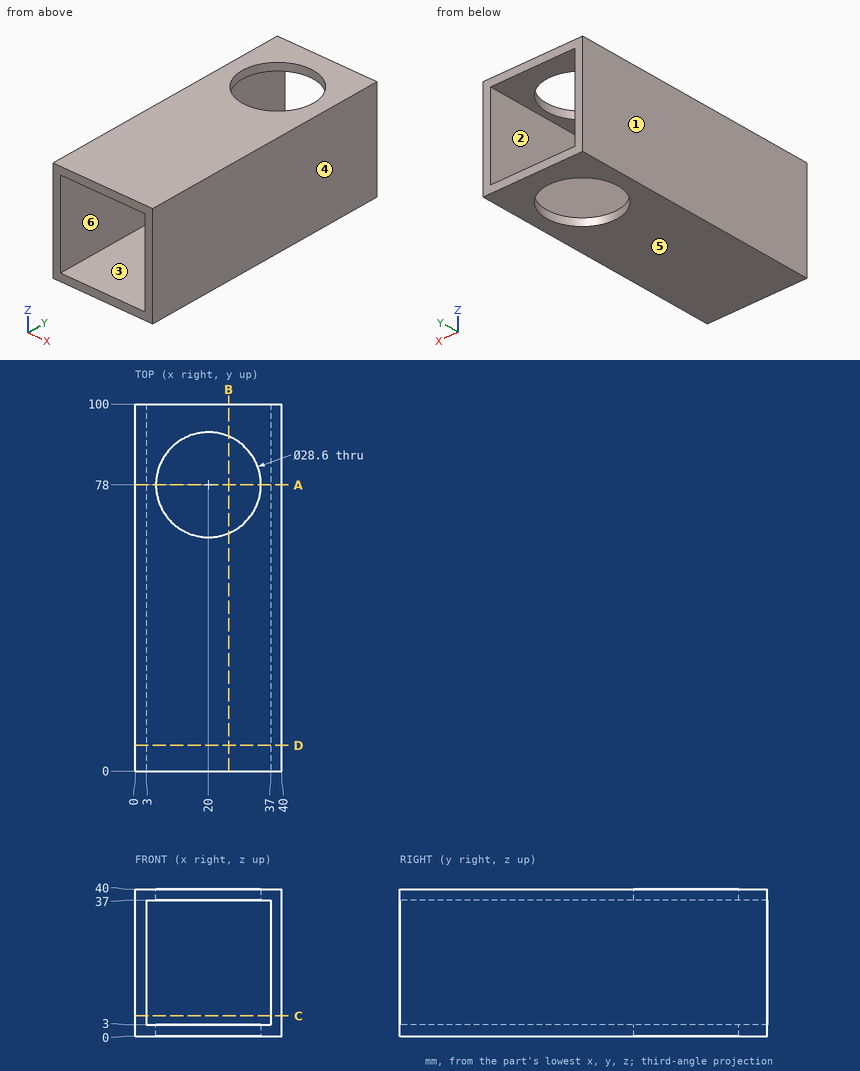
Check sheet for the drawn part. Datum: minimum x, y, z corner. Units: mm. A direction names the side the tool comes from. Round coordinates to 2 decimals unless told otherwise and drop trailing zeros. Order: outer loops, then holes, each group sorted by start corner. A loop starts at its lowest first (then second) coordinate and runs counter-clockwise, first axis right, second up.
1) Section check A-A (y = 78). Record the boundary of the cut face in (x, z), and give its area (3 significant figures).
2) Section check C-C (z = 5.5). Record the boundary of the cut face in (x, y).
3) Section check B-B (x = 25.5). Record the boundary of the cut face in (y, z).
4) Scan lines: line 1 (Z direction, x = 25, y = 96); line 2 (Y direction, x = 20, z = 1.6). Record each from-to range of solid material in increasing order.
5) Mould release check, pull along X, two halves, no side actions. Record for the marked faces 1, 2, 3 and 4: +X half, -X half, draft (parallel to the pull), parting line (faces both ways), or undercut.
6) Tool access check on the marked faces 5 and 6. Record the directions out of +Z, -Z, +X, -X, +Y, -Y that give a thin tool (end or side, any length) a straight path to the whole face; none if there is none.
7) Section check D-D (y = 7). Record the boundary of the cut face in (x, z), and give its area (3 significant figures).
Result:
1. outline: (0, 0) - (5.7, 0) - (5.7, 3) - (3, 3) - (3, 37) - (5.7, 37) - (5.7, 40) - (0, 40) - close; (34.3, 0) - (40, 0) - (40, 40) - (34.3, 40) - (34.3, 37) - (37, 37) - (37, 3) - (34.3, 3) - close
1. area: 272 mm2
2. outline: (0, 0) - (3, 0) - (3, 100) - (0, 100) - close; (37, 0) - (40, 0) - (40, 100) - (37, 100) - close
3. outline: (0, 0) - (64.8, 0) - (64.8, 3) - (0, 3) - close; (0, 37) - (64.8, 37) - (64.8, 40) - (0, 40) - close; (91.2, 0) - (100, 0) - (100, 3) - (91.2, 3) - close; (91.2, 37) - (100, 37) - (100, 40) - (91.2, 40) - close
4. line 1: z = 0 to 3, 37 to 40
4. line 2: y = 0 to 63.7, 92.3 to 100
5. face 1: -X half
5. face 2: undercut
5. face 3: undercut
5. face 4: +X half
6. face 5: -Z, +X, -X, +Y, -Y
6. face 6: +Y, -Y
7. outline: (0, 0) - (40, 0) - (40, 40) - (0, 40) - close; hole (3, 3) - (37, 3) - (37, 37) - (3, 37) - close
7. area: 444 mm2
